The drawing under review shows one solid part. Ordinate dimensions are in mm from its lowest x, y, z. A direction names the side the tool comes from. Round coordinates to 2 decimals unless told otherwise and drop trailing zeros. Write each loop counter-clockwise with the first axis right and the second up, starting at its lowest first coordinate (ties: lowest second). Pieces come first, ordered by that corner, then holes. Notation, with made-up numbers: M 6.25,3.25 L 16.25,3.25 A27 cw 16.25,36.25 Z; hole C -5,87.5 d9. An arc over 180 degrees is marked long. One line per item, written item: value. Start each with the question number.
1) Wall thickness on probe 1 along X at (y, z) = (1, 8); probe 2 along X at (y, z) = (2.6, 0.75); probe 3 along Z at (x, y) = (2, 2.1): over which ranges is each line inside the solid? List them lowest first.
2) Mouldability with a two-part tool opening along Z and no side actions: class the marked faces 4, 5, 6 and 7 as +Z half, -Z half, draft (parallel to the pull), parting line (faces both ways), or undercut.
3) Take a section at D-D, the plane x = 7.5. Write out the cut boundary in (y, z).
4) Take a section at B-B, the plane z = 1. Write out the cut boundary in (x, y).
5) Take a section at A-A, the plane x = 32.5. Write out the cut boundary in (y, z).
6) For P1, Ø0.9, axis at x = 32, y = 2, coming from the -Z side, flat-tipped, find the tip position at first contact; note if it passes through.
7) Tool access review of the marked faces 1, 2 and 3: name each direction out of +Z, -Z, +X, -X, +Y, -Y from which nothing blocks a thin tool from reaching the whole face with its end or side.
8) Take a section at C-C, the plane y = 2.7. State how many separate pieces and enclosed holes the cut face has.
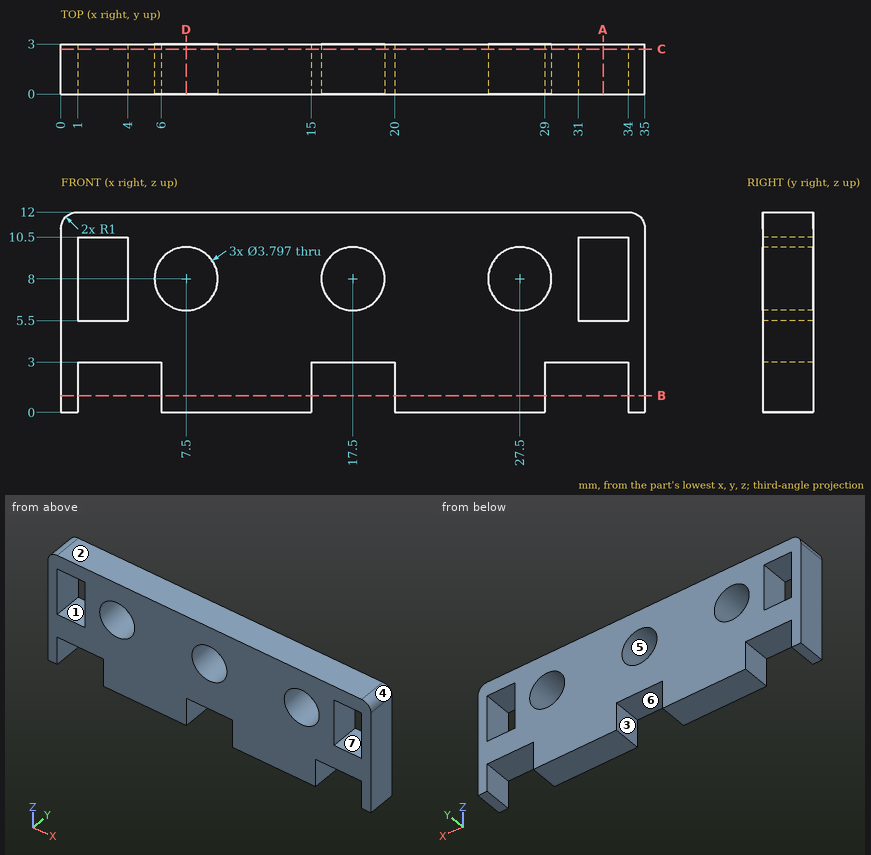
Checked values:
1. probe 1: x = 0 to 1, 4 to 5.6, 9.4 to 15.6, 19.4 to 25.6, 29.4 to 31, 34 to 35
1. probe 2: x = 0 to 1, 6 to 15, 20 to 29, 34 to 35
1. probe 3: z = 3 to 5.5, 10.5 to 12
2. face 4: +Z half
2. face 5: undercut
2. face 6: -Z half
2. face 7: undercut
3. outline: M 0,0 L 3,0 L 3,6.1 L 0,6.1 Z; M 0,9.9 L 3,9.9 L 3,12 L 0,12 Z
4. outline: M 0,0 L 1,0 L 1,3 L 0,3 Z; M 6,0 L 15,0 L 15,3 L 6,3 Z; M 20,0 L 29,0 L 29,3 L 20,3 Z; M 34,0 L 35,0 L 35,3 L 34,3 Z
5. outline: M 0,3 L 3,3 L 3,5.5 L 0,5.5 Z; M 0,10.5 L 3,10.5 L 3,12 L 0,12 Z
6. P1: stops at z = 3
7. face 1: +Y, -Y
7. face 2: +Z, +X, -X, +Y, -Y
7. face 3: -Z, +Y, -Y
8. separate pieces: 1
8. enclosed holes: 5
